Read the model definition and answer for the solid it produces. Units are mm, in the model's axes. A direction names the side the tool comes from. Give positions to 0.01 mm unless a question says otherwise; leave off trailing zeros. Loops run counter-clockwise (first coordinate to the right, second up) from the corner with the lowest first, then second, coordinate; pieces in that order, holes last. Notation, with made-up numbers: (-30, 31.5) - (-17, 31.5) arc R17 ccw to (-17, 54.5) - close; hole circle Ø1 at (37.25, 22). An arc over 180 degrees is marked (long way). Write item = value, one per line. Start each with the question number.
from build123d import *

# Parameters (mm, degrees)
SKETCH1_W           = 40.745918
SKETCH1_H           = 40
BOSS_EXTRUDE1_DEPTH = 20
FILLET1_R           = 1
SKETCH2_R           = 4
BOSS_EXTRUDE2_DEPTH = 6
SKETCH3_W           = 5
SKETCH3_H           = 8
CUT_EXTRUDE1_DEPTH  = 5
SKETCH4_R           = 4
BOSS_EXTRUDE3_DEPTH = 7
SKETCH5_R           = 1
CUT_EXTRUDE2_DEPTH  = 5
SKETCH6_R           = 1
CUT_EXTRUDE3_DEPTH  = 5


with BuildPart() as part:
    # Sketch1 → Boss-Extrude1 (new body)
    with BuildSketch(Plane.XY):
        with Locations((20.372959, 20)):
            Rectangle(SKETCH1_W, SKETCH1_H)
    extrude(amount=BOSS_EXTRUDE1_DEPTH)

    # Fillet1
    fillet1_edges = [part.edges().sort_by_distance(p)[0] for p in [
        (40.745918, 20, 20),
        (20.372959, 40, 20),
        (0, 20, 20),
        (20.372959, 40, 0),
        (40.745918, 20, 0),
        (20.372959, 0, 0),
        (0, 20, 0),
        (20.372959, 0, 20),
        (0, 40, 10),
        (40.745918, 40, 10),
        (40.745918, 0, 10),
        (0, 0, 10),
    ]]
    fillet(fillet1_edges, radius=FILLET1_R)

    # Sketch2 → Boss-Extrude2 (add)
    with BuildSketch(Plane(origin=(40.745918, 0, 0), x_dir=(0, 0, -1), z_dir=(1, 0, 0))):
        with Locations((-10, 30)):
            Circle(SKETCH2_R)
    extrude(amount=BOSS_EXTRUDE2_DEPTH)

    # Sketch3 → Cut-Extrude1 (cut)
    with BuildSketch(Plane(origin=(0, 40, 0), x_dir=(1, 0, 0), z_dir=(0, 1, 0))):
        with Locations((32.245918, -10)):
            Rectangle(SKETCH3_W, SKETCH3_H)
    extrude(amount=-CUT_EXTRUDE1_DEPTH, mode=Mode.SUBTRACT)

    # Sketch4 → Boss-Extrude3 (add)
    with BuildSketch(Plane.ZY):
        with Locations((10, 30)):
            Circle(SKETCH4_R)
    extrude(amount=BOSS_EXTRUDE3_DEPTH)

    # Sketch5 → Cut-Extrude2 (cut)
    with BuildSketch(Plane(origin=(40.745918, 0, 0), x_dir=(0, 0, -1), z_dir=(1, 0, 0))):
        with Locations((-17.5, 17.5)):
            Circle(SKETCH5_R)
        with Locations((-2.5, 17.5)):
            Circle(SKETCH5_R)
        with Locations((-2.5, 2.5)):
            Circle(SKETCH5_R)
        with Locations((-17.5, 2.5)):
            Circle(SKETCH5_R)
    extrude(amount=-CUT_EXTRUDE2_DEPTH, mode=Mode.SUBTRACT)

    # Sketch6 → Cut-Extrude3 (cut)
    with BuildSketch(Plane.ZY):
        with Locations((17, 10)):
            Circle(SKETCH6_R)
        with Locations((10, 3)):
            Circle(SKETCH6_R)
        with Locations((3, 10)):
            Circle(SKETCH6_R)
    extrude(amount=-CUT_EXTRUDE3_DEPTH, mode=Mode.SUBTRACT)


solid = part.part
1. A tool of negligible diameter and unlimited length cuts with its end or side. For faces 1 (the cylindrical face through (2.465, 3.676, 9.263)), 2 (the flat face through (35.746, 3, 18)), 3 (the flat face through (29.746, 38, 10)), from which of +Z, -Z, +X, -X, +Y, -Y can it reach the whole face along a straight path? Write none if from no direction.
2. Given P1, Ø1, axis at y = 10, z = 17, coming from the -X side; P2, Ø5, axis at y = 11.5, z = 9.5, coming from the -X side; P3, Ø1.6, axis at y = 2.5, z = 17.5, coming from the +X side, each flat-ended and moving along its own axis, determine where each tip first touches the part or whether it passes through.
3. A cutting plane is placed at A-A on y = 15.5. Give the vertices of the cut face in (x, z).
4. Consider line 1 along Y through (x, z) = (37.75, 17.5); line 2 along X through (y, z) = (36, 10); line 3 along Y through (x, z) = (1.5, 3). Determine where each line is inside the solid, lowest interval first. Write a range as [from, to].
5. For a pull along Y with two mould halves and no side action, classify faces 4 (the cylindrical face through (2, 11, 3)), 5 (the flat face through (20, 40, 10)), 6 (the cylindrical face through (38.281, 16.524, 2.717)), 7 (the flat face through (46.746, 30, 10)) as released by +Y, released by -Y, zero draft, split by the parting line, or undercut.
6. A cutting plane is placed at C-C on y = 32. Give the vertices of the cut face in (x, z).
7. A cutting plane is placed at B-B on x = -2. Give the vertices of the cut face in (y, z), and give its area (3 significant figures).
Reply:
q1.face_1 = -X
q1.face_2 = +X
q1.face_3 = +Y
q2.P1 = 5
q2.P2 = 0
q2.P3 = 35.75
q3.outline = (0, 1) arc R1 ccw to (1, 0) - (39.75, 0) arc R1 ccw to (40.75, 1) - (40.75, 19) arc R1 ccw to (39.75, 20) - (1, 20) arc R1 ccw to (0, 19) - close
q4.line_1 = [0, 1.5], [3.5, 16.5], [18.5, 40]
q4.line_2 = [0, 29.75], [34.75, 40.75]
q4.line_3 = [0, 9], [11, 40]
q5.face_4 = undercut
q5.face_5 = released by +Y
q5.face_6 = undercut
q5.face_7 = zero draft
q6.outline = (-7, 6.54) - (0, 6.54) - (0, 1) arc R1 ccw to (1, 0) - (39.75, 0) arc R1 ccw to (40.75, 1) - (40.75, 6.54) - (46.75, 6.54) - (46.75, 13.46) - (40.75, 13.46) - (40.75, 19) arc R1 ccw to (39.75, 20) - (1, 20) arc R1 ccw to (0, 19) - (0, 13.46) - (-7, 13.46) - close
q7.outline = circle Ø8 at (30, 10)
q7.area = 50.3 mm^2
